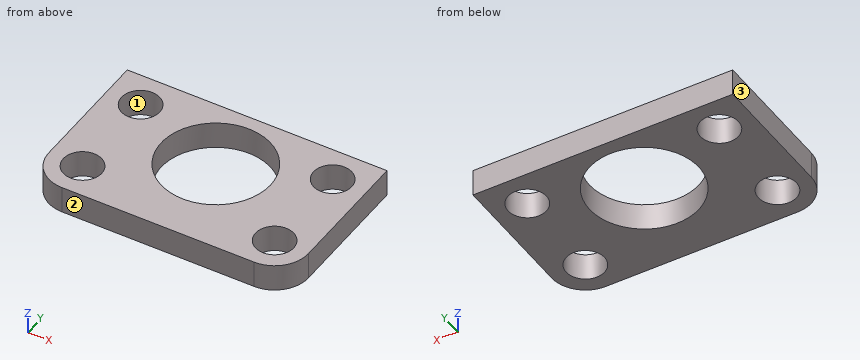
```python
from build123d import *

# Parameters (mm, degrees)
F0_W     = 30.477764
F0_H     = 19.177
F0_R     = 2.2479
F0_R_2   = 6.4135
F1_DEPTH = 3.175
F2_R     = 3.96875


with BuildPart() as f1:
    # F0 (on Top) → F1 (new body)
    with BuildSketch(Plane.XY):
        with Locations((15.238882, -9.5885)):
            Rectangle(F0_W, F0_H)
        with Locations((3.96875, -15.20825)):
            Circle(F0_R, mode=Mode.SUBTRACT)
        with Locations((26.509014, -15.20825)):
            Circle(F0_R, mode=Mode.SUBTRACT)
        with Locations((3.96875, -3.96875)):
            Circle(F0_R, mode=Mode.SUBTRACT)
        with Locations((15.238882, -8.001)):
            Circle(F0_R_2, mode=Mode.SUBTRACT)
        with Locations((26.509014, -3.96875)):
            Circle(F0_R, mode=Mode.SUBTRACT)
    extrude(amount=F1_DEPTH)

    # F2
    f2_edges = [f1.edges().sort_by_distance(p)[0] for p in [
        (0, -19.177, 1.5875),
        (30.477764, -19.177, 1.5875),
    ]]
    fillet(f2_edges, radius=F2_R)


solid = f1.part
```
Can you work these out from the model? Positions are in its coordinate system, mm. Face numbers are marked on the shaded views. Give positions to 0.01 mm unless a question says otherwise; leave off trailing zeros. Write each loop counter-clockwise with the first axis right and the second up, starting at its lowest first coordinate (ties: lowest second). Pieces come first, ordered by that corner, then holes. Notation, with made-up numbers: (83.25, 1) -> (110.25, 1) arc R21 cw to (110.25, 21) -> close; hole circle Ø10 at (80.5, 38). An arc over 180 degrees is marked (long way). Write item = value, one per line.
(1) Thinking about a two-plate mould opening in X: for the marked faces 1, 2 and 3, which applies, released by +X, released by -X, zero draft, split by the parting line, or undercut?
Worked out:
face_1 = undercut
face_2 = zero draft
face_3 = released by -X
(2) Suppose I cut it at C-C on x = 16.5. Write out the boundary of the cut face in (y, z) (3 decimals).
Worked out:
outline = (-19.177, 0) -> (-14.289, 0) -> (-14.289, 3.175) -> (-19.177, 3.175) -> close; (-1.713, 0) -> (0, 0) -> (0, 3.175) -> (-1.713, 3.175) -> close
(3) Suppose I cut it at A-A on y = -5.25. Write out the boundary of the cut face in (x, z) (3 decimals).
Worked out:
outline = (0, 0) -> (2.122, 0) -> (2.122, 3.175) -> (0, 3.175) -> close; (5.816, 0) -> (9.445, 0) -> (9.445, 3.175) -> (5.816, 3.175) -> close; (21.032, 0) -> (24.662, 0) -> (24.662, 3.175) -> (21.032, 3.175) -> close; (28.356, 0) -> (30.478, 0) -> (30.478, 3.175) -> (28.356, 3.175) -> close
(4) I need wall thicknesses on probe 1 along Y at (x, z) = (4, 0.7); probe 2 along X at (y, z) = (-15.25, 0.9); probe 3 along Y at (x, z) = (24.5, 1.05). Which ranges of each line are inside material? Lowest first, please. Write a range as from..to.
Worked out:
probe_1 = -19.18..-17.46, -12.96..-6.22, -1.72..0
probe_2 = 0..1.72, 6.22..24.26, 28.76..30.48
probe_3 = -19.18..-16.22, -14.2..-4.98, -2.96..0
(5) Suppose I cut it at D-D on z = 0.85. Write out the boundary of the cut face in (x, y), then the cut area to 3 significant figures.
Worked out:
outline = (0, -15.21) arc R3.97 ccw to (3.97, -19.18) -> (26.51, -19.18) arc R3.97 ccw to (30.48, -15.21) -> (30.48, 0) -> (0, 0) -> close; hole circle Ø4.5 at (3.97, -15.21); hole circle Ø4.5 at (3.97, -3.97); hole circle Ø12.83 at (15.24, -8); hole circle Ø4.5 at (26.51, -15.21); hole circle Ø4.5 at (26.51, -3.97)
area = 385 mm^2
(6) Suppose I cut it at B-B on x = 25.5. Write out the boundary of the cut face in (y, z) (3 decimals).
Worked out:
outline = (-19.177, 0) -> (-17.217, 0) -> (-17.217, 3.175) -> (-19.177, 3.175) -> close; (-13.2, 0) -> (-5.977, 0) -> (-5.977, 3.175) -> (-13.2, 3.175) -> close; (-1.96, 0) -> (0, 0) -> (0, 3.175) -> (-1.96, 3.175) -> close
